CAD build for the part. Positions are in the model's coordinates, mm. Face numbers are marked on the shaded views. A direction names the side the tool comes from. Round coordinates to 2 decimals unless told otherwise and drop trailing zeros. Write each loop counter-clockwise with the first axis right and the second up, starting at its lowest first coordinate (ties: lowest second). Pieces come first, ordered by that corner, then holes. Notation, with made-up numbers: (19, 50) - (56, 50) arc R17 ccw to (56, 72) - close; hole circle Ø2 at (73, 44). An arc over 180 degrees is marked (long way). Answer in a Markdown table with one row per item.
```python
from build123d import *

# Parameters (mm, degrees)
SKETCH1_W           = 42
SKETCH1_H           = 42
BOSS_EXTRUDE1_DEPTH = 39.8
SKETCH2_R           = 10.95
BOSS_EXTRUDE2_DEPTH = 2
SKETCH3_R           = 1.25
CUT_EXTRUDE1_DEPTH  = 10
SKETCH4_R           = 2
BOSS_EXTRUDE3_DEPTH = 22


with BuildPart() as part:
    # Sketch1 → Boss-Extrude1 (new body)
    with BuildSketch(Plane.XY):
        Rectangle(SKETCH1_W, SKETCH1_H)
    extrude(amount=BOSS_EXTRUDE1_DEPTH)

    # Sketch2 → Boss-Extrude2 (add)
    with BuildSketch(Plane.XY.offset(39.8)):
        Circle(SKETCH2_R)
    extrude(amount=BOSS_EXTRUDE2_DEPTH)

    # Sketch3 → Cut-Extrude1 (cut)
    with BuildSketch(Plane.XY.offset(39.8)):
        with Locations((-17, 17)):
            Circle(SKETCH3_R)
        with Locations((17, 17)):
            Circle(SKETCH3_R)
        with Locations((17, -17)):
            Circle(SKETCH3_R)
        with Locations((-17, -17)):
            Circle(SKETCH3_R)
    extrude(amount=-CUT_EXTRUDE1_DEPTH, mode=Mode.SUBTRACT)

    # Sketch4 → Boss-Extrude3 (add)
    with BuildSketch(Plane.XY.offset(41.8)):
        Circle(SKETCH4_R)
    extrude(amount=BOSS_EXTRUDE3_DEPTH)


solid = part.part
```
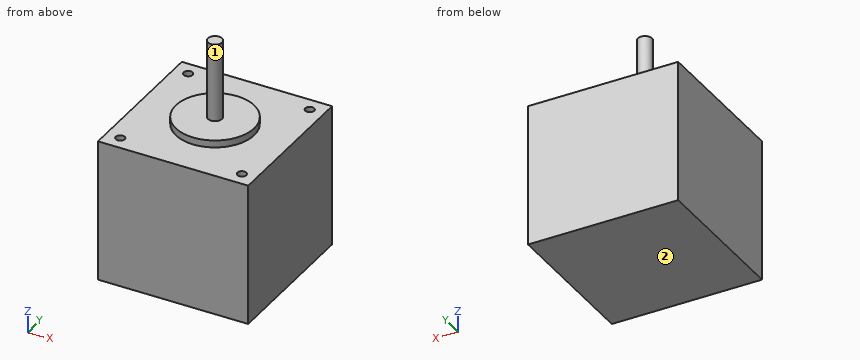
Q1. Saw through at B-B on y = -17. List the corners of the cut face in (x, z).
Computed:
| item | result |
|---|---|
| outline | (-21, 0) - (21, 0) - (21, 39.8) - (18.25, 39.8) - (18.25, 29.8) - (15.75, 29.8) - (15.75, 39.8) - (-15.75, 39.8) - (-15.75, 29.8) - (-18.25, 29.8) - (-18.25, 39.8) - (-21, 39.8) - close |
Q2. Saw through at D-D on y = -10. List the corners of the cut face in (x, z).
Computed:
| item | result |
|---|---|
| outline | (-21, 0) - (21, 0) - (21, 39.8) - (4.46, 39.8) - (4.46, 41.8) - (-4.46, 41.8) - (-4.46, 39.8) - (-21, 39.8) - close |
Q3. Drill centre lines: line 1 (Y direction, x = 17, z = 38); line 2 (Y direction, x = 16, z = 36.5); line 3 (Z direction, x = 2.5, y = 15.5). Where is each one in solid material? Low to high.
Computed:
| item | result |
|---|---|
| line 1 | y = -21 to -18.25, -15.75 to 15.75, 18.25 to 21 |
| line 2 | y = -21 to -17.75, -16.25 to 16.25, 17.75 to 21 |
| line 3 | z = 0 to 39.8 |
Q4. 3-axis set-ups, long thin cutter, end or side, ignore diameter. For the marked faces 1 and 2: which of +Z, -Z, +X, -X, +Y, -Y reach the whole face in a straight line?
Computed:
| item | result |
|---|---|
| face 1 | +Z |
| face 2 | -Z, +X, -X, +Y, -Y |
Q5. Flat gauge pins, fed straight in: pin 1 (1.5 mm diameter, centred on x = 17, y = 17, fed in from +Z); pin 2 (6 mm diameter, centred on x = 12, y = 4, fed in from +Z); pin 3 (2 mm diameter, centred on x = -16.5, y = 16.5, fed in from +Z). Where does each tip first touch, or does it go through?
Computed:
| item | result |
|---|---|
| pin 1 | stops at z = 29.8 |
| pin 2 | stops at z = 41.8 |
| pin 3 | stops at z = 39.8 |
Q6. Saw through at C-C on z = 60. List the corners of the cut face in (x, y), then the cut area to 3 significant figures.
Computed:
| item | result |
|---|---|
| outline | circle Ø4 at (0, 0) |
| area | 12.6 mm2 |
Q7. Saw through at A-A on x = 0. List the corners of the cut face in (y, z), then the cut area to 3 significant figures.
Computed:
| item | result |
|---|---|
| outline | (-21, 0) - (21, 0) - (21, 39.8) - (10.95, 39.8) - (10.95, 41.8) - (2, 41.8) - (2, 63.8) - (-2, 63.8) - (-2, 41.8) - (-10.95, 41.8) - (-10.95, 39.8) - (-21, 39.8) - close |
| area | 1,800 mm2 |
